from build123d import *

# Parameters (mm, degrees)
F1_DEPTH    = 20
F2_W        = 6
F2_H        = 15
F3_DEPTH    = 20.001
F4_T1_DEPTH = 37.1421356237
F5_W        = 20
F5_H        = 20
F5_W_2      = 18
F5_H_2      = 18
F6_DEPTH    = 1.5


# Not quite as in the source:
# - a fillet or chamfer that OpenCascade refuses, or shapes differently, is made with other operations: its cross-section is extruded or revolved along the edge and cut away or added


with BuildPart() as f1:
    # F0 (on Right) → F1 (new body)
    with BuildSketch(Plane.YZ):
        with BuildLine():
            Line((-18.178238757, 7.9620768987), (-18.178238757, 4.9620768987))
            Line((-18.178238757, 4.9620768987), (1.821761243, 4.9620768987))
            Line((1.821761243, 4.9620768987), (1.821761243, 7.9620768987))
            Line((1.821761243, 7.9620768987), (-5.678238757, 7.9620768987))
            Line((-5.678238757, 7.9620768987), (-5.678238757, 9.3611253762))
            ThreePointArc((-5.678238757, 9.3611253762), (-5.2512465802, 11.5609410366), (-4.321354907, 13.5997673497))
            ThreePointArc((-4.321354907, 13.5997673497), (-1.7002475397, 16.4152583597), (1.821761243, 17.9620768987))
            Line((1.821761243, 17.9620768987), (1.821761243, 22.9620768987))
            Line((1.821761243, 22.9620768987), (-18.178238757, 7.9620768987))
        make_face()
    extrude(amount=F1_DEPTH)

    # F2 (on face) → F3 (cut, through all)
    with BuildSketch(Plane(origin=(0, 1.821761243, 0), x_dir=(-1, 0, 0), z_dir=(0, 1, 0))):
        with Locations((-17, 15.4620768987)):
            Rectangle(F2_W, F2_H)
        with Locations((-3, 15.4620768987)):
            Rectangle(F2_W, F2_H)
    extrude(amount=-F3_DEPTH, mode=Mode.SUBTRACT)

    # F4: fillet of radius 3 on 1 edges, made by hand

    # F4_s2 → F4_t1 (cut)
    with BuildSketch(Plane.YZ.offset(-8.5710678119)):
        with BuildLine():
            ThreePointArc((-2.8409804568, 19.4650206238), (-0.1206191471, 19.9203551155), (1.821761243, 17.9620768987))
            Line((1.821761243, 17.9620768987), (1.821761243, 22.9620768987))
            Line((1.821761243, 22.9620768987), (-2.8409804568, 19.4650206238))
        make_face()
    extrude(amount=F4_T1_DEPTH, mode=Mode.SUBTRACT)

    # F5 (on face) → F6 (join)
    with BuildSketch(Plane(origin=(0, 0, 4.9620768987), x_dir=(1, 0, 0), z_dir=(0, 0, -1))):
        with Locations((10, 8.178238757)):
            Rectangle(F5_W, F5_H)
        with Locations((10, 8.178238757)):
            Rectangle(F5_W_2, F5_H_2, mode=Mode.SUBTRACT)
    extrude(amount=F6_DEPTH)


solid = f1.part
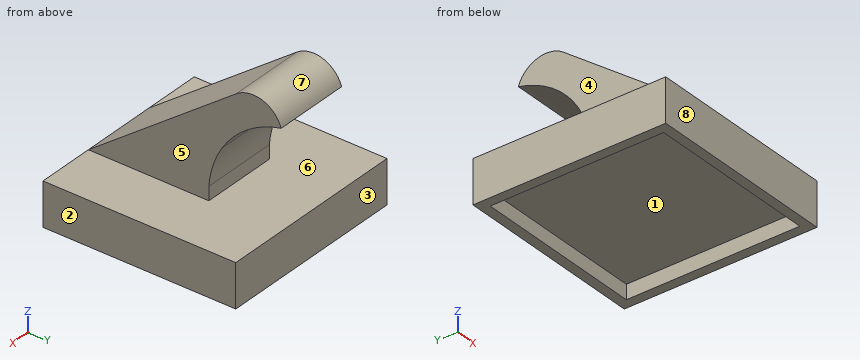
Could you check a few things on this model? Use its own coordinates, in mm. Face numbers are marked on the shaded views. A direction names the side the tool comes from. Give positions to 0.01 mm unless a question says otherwise; leave off trailing zeros. Order: outer loops, then holes, each group sorted by start corner. A loop starts at its lowest first (then second) coordinate and runs counter-clockwise, first axis right, second up. Notation, with made-up numbers: (85.25, 0.5) -> (134.25, 0.5) arc R6 cw to (134.25, 7.5) -> close; hole circle Ø3 at (-33.75, 2.25). An arc over 180 degrees is marked (long way). Answer in a Markdown table with one row per item. Add a question column.
Item 1: Imagine slicing it at D-D (z = 15). List the corners of the cut face in (x, y) for me, and give its area (3 significant figures).
Item 2: Imagine slicing it at A-A (y = -2.5). List the corners of the cut face in (x, z) for me.
Item 3: We'd pull the mould along Z, two halves only. Please class the marked faces 6, 7 and 8: pulls with the +Z half, pulls with the -Z half, needs draft (parallel to the pull), parting line crosses it, or undercut.
Item 4: Imagine slicing it at C-C (y = -13.75). List the corners of the cut face in (x, z) for me, and give its area (3 significant figures).
Item 5: Imagine slicing it at B-B (x = 3.75). List the corners of the cut face in (y, z) for me, and give its area (3 significant figures).
Item 6: I'm going to push flat-ended pins straight in: P1, Ø6, axis at y = -4, z = 13, coming from the -X side; P2, Ø12, axis at x = 6, y = -11.5, coming from the +Z side; P3, Ø1.5, axis at x = 9, y = -5, coming from the -Z side; P4, Ø5, axis at y = -15.5, z = 9, coming from the +X side. Where does each tip first touch, or does it pass through?
Item 7: Please list where these lines run through material, in increasing order: probe 1 along X at (y, z) = (-14.75, 10.5); probe 2 along Z at (x, y) = (14.5, -2.5); probe 3 along Z at (x, y) = (9.25, -12.75).
Item 8: For the marked faces 1, 2, 3, 4 and 5, which set-ups out of +Z, -Z, +X, -X, +Y, -Y let a thin tool reach every point of the face, with its end or its side?
Result:
| question | item | result |
|---|---|---|
| 1 | outline | (6, -8.79) -> (14, -8.79) -> (14, -3.28) -> (6, -3.28) -> close |
| 1 | area | 44.1 mm2 |
| 2 | outline | (0, 3.46) -> (1, 3.46) -> (1, 4.96) -> (19, 4.96) -> (19, 3.46) -> (20, 3.46) -> (20, 7.96) -> (0, 7.96) -> close; (6, 15.78) -> (14, 15.78) -> (14, 19.69) -> (6, 19.69) -> close |
| 3 | face 6 | undercut |
| 3 | face 7 | pulls with the +Z half |
| 3 | face 8 | needs draft |
| 4 | outline | (0, 3.46) -> (1, 3.46) -> (1, 4.96) -> (19, 4.96) -> (19, 3.46) -> (20, 3.46) -> (20, 7.96) -> (14, 7.96) -> (14, 11.28) -> (6, 11.28) -> (6, 7.96) -> (0, 7.96) -> close |
| 4 | area | 89.6 mm2 |
| 5 | outline | (-18.18, 3.46) -> (-17.18, 3.46) -> (-17.18, 4.96) -> (0.82, 4.96) -> (0.82, 3.46) -> (1.82, 3.46) -> (1.82, 7.96) -> (-18.18, 7.96) -> close |
| 5 | area | 63.0 mm2 |
| 6 | P1 | x = 6 |
| 6 | P2 | z = 17.47 |
| 6 | P3 | z = 4.96 |
| 6 | P4 | x = 20 |
| 7 | probe 1 | 6 to 14 |
| 7 | probe 2 | 4.96 to 7.96 |
| 7 | probe 3 | 4.96 to 12.03 |
| 8 | face 1 | -Z |
| 8 | face 2 | +Z, -Z, +X, +Y, -Y |
| 8 | face 3 | +Z, -Z, +X, -X, +Y |
| 8 | face 4 | +Z, -X, +Y, -Y |
| 8 | face 5 | +Z, +X, +Y, -Y |
